Geometry check sheet. Reference: the model listing, model coordinates, mm. Give positions to 0.01 mm unless a question says otherwise; leave off trailing zeros. Write each loop counter-clockwise with the first axis right and the second up, starting at its lowest first coordinate (ties: lowest second). Pieces come first, ordered by that corner, then holes. Notation, with made-up numbers: (65, 33) -> (86, 33) arc R20 cw to (86, 64) -> close; hole circle Ø1 at (-20, -33.5). An arc over 180 degrees is marked (long way). Write item = value, one per line. Start each with the question number.
1. Cross-section at D-D, the plane z = 63.5. Record the cut outline in (x, y).
2. Cross-section at B-B, the plane z = 8. Record the cut outline in (x, y), plus the area to 3 significant figures.
3. Mould release check, pull along Z, two halves, no side actions. Record for faces 1 (the cylindrical face through (-42.594, 4.19, -55.55)), 2 (the conical face through (-1, 6.22, -61.08)), 3 (the flat face through (-57, 8.5, 10)): pulls with the +Z half, pulls with the -Z half, needs draft (parallel to the pull), parting line crosses it, or undercut.
4. Thickness scan on line 1 along X through (y, z) = (3.25, 0); line 2 along Z through (x, y) = (63.5, 2); line 3 along Z through (x, y) = (20, 3.25). Record the ranges inside material, lowest first.
5. Cross-section at C-C, the plane x = 46.5. Record the cut outline in (y, z), plus the area to 3 significant figures.
6. Depth check by flat-ended pin: P1, Ø4, axis at y = 2.5, z = -6.5, coming from the -X side; P2, Ø6.5, axis at x = 0, z = 63.5, coming from the -Y side; P3, Ø4, axis at y = 1.5, z = 41, coming from the -X side; P4, Ø3, axis at y = 7, z = 13, coming from the -X side. Enter the tip coordinate at first touch or a pass-through.
7. Cross-section at A-A, the plane y = 4.5. Record the cut outline in (x, z), plus the area to 3 significant figures.
```python
from build123d import *

# Parameters (mm, degrees)
SKETCH_1_R               = 70
SKETCH_1_R_2             = 2.5
SKETCH_1_R_3             = 57.5
EXTRUDE_1_DEPTH          = 8.5
PATTERN_CIRCULAR_1_COUNT = 4


with BuildPart() as part:
    # Sketch 1 → Extrude 1 (new body)
    with BuildSketch(Plane(origin=(0, 0, 0), x_dir=(1, 0, 0), z_dir=(0, 1, 0))):
        with Locations(Location((0, 0, 0), (0, 0, 270))):
            Circle(SKETCH_1_R)
        with Locations(Location((-63.5, 0, 0), (0, 0, 270))):
            Circle(SKETCH_1_R_2, mode=Mode.SUBTRACT)
        with Locations(Location((0, -63.5, 0), (0, 0, 270))):
            Circle(SKETCH_1_R_2, mode=Mode.SUBTRACT)
        with Locations(Location((63.5, 0, 0), (0, 0, 270))):
            Circle(SKETCH_1_R_2, mode=Mode.SUBTRACT)
        with Locations(Location((0, 63.5, 0), (0, 0, 270))):
            Circle(SKETCH_1_R_2, mode=Mode.SUBTRACT)
        with Locations(Location((0, 0, 0), (0, 0, 270))):
            Circle(SKETCH_1_R_3, mode=Mode.SUBTRACT)
    extrude(amount=EXTRUDE_1_DEPTH)

    # Sketch 2 → Cut-Revolve 1 (revolve, cut)
    with BuildSketch(Plane.XY.offset(-63.5), mode=Mode.PRIVATE) as cut_revolve_1_sk:
        Polygon((0, 8.5), (4.9, 8.5), (1.6, 5.2), (0, 5.2), align=None)
    cut_revolve_1 = revolve(cut_revolve_1_sk.sketch.rotate(Axis((0, 0, -63.5), (0, 1, 0)), 270), axis=Axis((0, 0, -63.5), (0, 1, 0)), mode=Mode.SUBTRACT)

    # Pattern Circular 1: Cut-Revolve 1 ×4 about axis
    pattern_circular_1_axis = Axis((0, 0, 0), (0, 1, 0))
    for i in range(1, PATTERN_CIRCULAR_1_COUNT):
        add(cut_revolve_1.rotate(pattern_circular_1_axis, i * 360 / PATTERN_CIRCULAR_1_COUNT), mode=Mode.SUBTRACT)


solid = part.part
```
Answers:
q1.outline = (-29.46, 0) -> (-2.5, 0) -> (-2.5, 6.1) -> (-4.9, 8.5) -> (-29.46, 8.5) -> close; (2.5, 0) -> (29.46, 0) -> (29.46, 8.5) -> (4.9, 8.5) -> (2.5, 6.1) -> close
q2.outline = (-69.54, 0) -> (-56.94, 0) -> (-56.94, 8.5) -> (-69.54, 8.5) -> close; (56.94, 0) -> (69.54, 0) -> (69.54, 8.5) -> (56.94, 8.5) -> close
q2.area = 214 mm^2
q3.face_1 = parting line crosses it
q3.face_2 = undercut
q3.face_3 = needs draft
q4.line_1 = -70 to -66, -61 to -57.5, 57.5 to 61, 66 to 70
q4.line_2 = -29.46 to -2.5, 2.5 to 29.46
q4.line_3 = -67.08 to -53.91, 53.91 to 67.08
q5.outline = (0, -52.32) -> (8.5, -52.32) -> (8.5, -33.82) -> (0, -33.82) -> close; (0, 33.82) -> (8.5, 33.82) -> (8.5, 52.32) -> (0, 52.32) -> close
q5.area = 315 mm^2
q6.P1 = -69.86
q6.P2 = 0
q6.P3 = -58.13
q6.P4 = -69.05
q7.outline = circle Ø140 at (0, 0); hole circle Ø5 at (-63.5, 0); hole circle Ø115 at (0, 0); hole circle Ø5 at (0, -63.5); hole circle Ø5 at (0, 63.5); hole circle Ø5 at (63.5, 0)
q7.area = 4,930 mm^2
